```python
from build123d import *

# Parameters (mm, degrees)
SKETCH1_W           = 10
SKETCH1_H           = 10
BOSS_EXTRUDE1_DEPTH = 2.5
SKETCH2_R           = 0.75
SKETCH2_R_2         = 1
SKETCH2_R_3         = 1.25
SKETCH2_R_4         = 1.5
CUT_EXTRUDE1_DEPTH  = 24.468063405


with BuildPart() as part:
    # Sketch1 → Boss-Extrude1 (new body)
    with BuildSketch(Plane(origin=(0, 0, 0), x_dir=(1, 0, 0), z_dir=(0, 1, 0))):
        Rectangle(SKETCH1_W, SKETCH1_H)
        with BuildLine():
            Line((-5, -5), (-5, 5))
            Line((-5, 5), (-14.671400751, 5))
            ThreePointArc((-14.671400751, 5), (-15.5, 0), (-14.671400751, -5))
            Line((-14.671400751, -5), (-5, -5))
        make_face()
        with BuildLine():
            Line((-14.671400751, 5), (-5, 5))
            Line((-5, 5), (-5, 14.671400751))
            ThreePointArc((-5, 14.671400751), (-10.960155108, 10.960155108), (-14.671400751, 5))
        make_face()
        with BuildLine():
            Line((-5, 5), (5, 5))
            Line((5, 5), (5, 14.671400751))
            ThreePointArc((5, 14.671400751), (0, 15.5), (-5, 14.671400751))
            Line((-5, 14.671400751), (-5, 5))
        make_face()
        with BuildLine():
            Line((5, 5), (14.671400751, 5))
            ThreePointArc((14.671400751, 5), (10.960155108, 10.960155108), (5, 14.671400751))
            Line((5, 14.671400751), (5, 5))
        make_face()
        with BuildLine():
            ThreePointArc((15.5, 0), (15.291447146, 2.534096324), (14.671400751, 5))
            Line((14.671400751, 5), (5, 5))
            Line((5, 5), (5, -5))
            Line((5, -5), (14.671400751, -5))
            ThreePointArc((14.671400751, -5), (15.291447146, -2.534096324), (15.5, 0))
        make_face()
        with BuildLine():
            Line((16.5, -5), (16.5, 5))
            Line((16.5, 5), (14.671400751, 5))
            ThreePointArc((14.671400751, 5), (15.291447146, 2.534096324), (15.5, 0))
            ThreePointArc((15.5, 0), (15.291447146, -2.534096324), (14.671400751, -5))
            Line((14.671400751, -5), (16.5, -5))
        make_face()
        with BuildLine():
            ThreePointArc((5, -14.671400751), (10.960155108, -10.960155108), (14.671400751, -5))
            Line((14.671400751, -5), (5, -5))
            Line((5, -5), (5, -14.671400751))
        make_face()
        with BuildLine():
            Line((5, -14.671400751), (5, -5))
            Line((5, -5), (-5, -5))
            Line((-5, -5), (-5, -14.671400751))
            ThreePointArc((-5, -14.671400751), (0, -15.5), (5, -14.671400751))
        make_face()
        with BuildLine():
            Line((-5, -14.671400751), (-5, -5))
            Line((-5, -5), (-14.671400751, -5))
            ThreePointArc((-14.671400751, -5), (-10.960155108, -10.960155108), (-5, -14.671400751))
        make_face()
        with BuildLine():
            ThreePointArc((-14.671400751, -5), (-15.5, 0), (-14.671400751, 5))
            Line((-14.671400751, 5), (-16.5, 5))
            Line((-16.5, 5), (-16.5, -5))
            Line((-16.5, -5), (-14.671400751, -5))
        make_face()
        with BuildLine():
            Line((5, -16.5), (5, -14.671400751))
            ThreePointArc((5, -14.671400751), (0, -15.5), (-5, -14.671400751))
            Line((-5, -14.671400751), (-5, -16.5))
            Line((-5, -16.5), (5, -16.5))
        make_face()
        with BuildLine():
            ThreePointArc((-5, 14.671400751), (0, 15.5), (5, 14.671400751))
            Line((5, 14.671400751), (5, 16.5))
            Line((5, 16.5), (-5, 16.5))
            Line((-5, 16.5), (-5, 14.671400751))
        make_face()
    extrude(amount=BOSS_EXTRUDE1_DEPTH)

    # Sketch2 → Cut-Extrude1 (cut, through all)
    with BuildSketch(Plane(origin=(0, 2.5, 0), x_dir=(1, 0, 0), z_dir=(0, 1, 0))):
        with Locations(Location((0, 0, 0), (0, 0, 270))):
            Circle(SKETCH2_R)
        with Locations(Location((0, 3.75, 0), (0, 0, 270))):
            Circle(SKETCH2_R_2)
        with Locations(Location((0, 8, 0), (0, 0, 270))):
            Circle(SKETCH2_R_3)
        with Locations(Location((0, 12.75, 0), (0, 0, 270))):
            Circle(SKETCH2_R_4)
        with Locations(Location((3.247595264, 1.875, 0), (0, 0, 270))):
            Circle(SKETCH2_R_2)
        with Locations(Location((3.247595264, -1.875, 0), (0, 0, 270))):
            Circle(SKETCH2_R_2)
        with Locations(Location((0, -3.75, 0), (0, 0, 270))):
            Circle(SKETCH2_R_2)
        with Locations(Location((-3.247595264, -1.875, 0), (0, 0, 270))):
            Circle(SKETCH2_R_2)
        with Locations(Location((-3.247595264, 1.875, 0), (0, 0, 270))):
            Circle(SKETCH2_R_2)
        with Locations(Location((4, 6.92820323, 0), (0, 0, 270))):
            Circle(SKETCH2_R_3)
        with Locations(Location((6.92820323, 4, 0), (0, 0, 270))):
            Circle(SKETCH2_R_3)
        with Locations(Location((8, 0, 0), (0, 0, 270))):
            Circle(SKETCH2_R_3)
        with Locations(Location((6.92820323, -4, 0), (0, 0, 270))):
            Circle(SKETCH2_R_3)
        with Locations(Location((4, -6.92820323, 0), (0, 0, 270))):
            Circle(SKETCH2_R_3)
        with Locations(Location((0, -8, 0), (0, 0, 270))):
            Circle(SKETCH2_R_3)
        with Locations(Location((-4, -6.92820323, 0), (0, 0, 270))):
            Circle(SKETCH2_R_3)
        with Locations(Location((-6.92820323, -4, 0), (0, 0, 270))):
            Circle(SKETCH2_R_3)
        with Locations(Location((-8, 0, 0), (0, 0, 270))):
            Circle(SKETCH2_R_3)
        with Locations(Location((-6.92820323, 4, 0), (0, 0, 270))):
            Circle(SKETCH2_R_3)
        with Locations(Location((-4, 6.92820323, 0), (0, 0, 270))):
            Circle(SKETCH2_R_3)
        with Locations(Location((4.879213763, 11.77946404, 0), (0, 0, 270))):
            Circle(SKETCH2_R_4)
        with Locations(Location((9.01561146, 9.01561146, 0), (0, 0, 270))):
            Circle(SKETCH2_R_4)
        with Locations(Location((11.77946404, 4.879213763, 0), (0, 0, 270))):
            Circle(SKETCH2_R_4)
        with Locations(Location((12.75, 0, 0), (0, 0, 270))):
            Circle(SKETCH2_R_4)
        with Locations(Location((11.77946404, -4.879213763, 0), (0, 0, 270))):
            Circle(SKETCH2_R_4)
        with Locations(Location((9.01561146, -9.01561146, 0), (0, 0, 270))):
            Circle(SKETCH2_R_4)
        with Locations(Location((4.879213763, -11.77946404, 0), (0, 0, 270))):
            Circle(SKETCH2_R_4)
        with Locations(Location((0, -12.75, 0), (0, 0, 270))):
            Circle(SKETCH2_R_4)
        with Locations(Location((-4.879213763, -11.77946404, 0), (0, 0, 270))):
            Circle(SKETCH2_R_4)
        with Locations(Location((-9.01561146, -9.01561146, 0), (0, 0, 270))):
            Circle(SKETCH2_R_4)
        with Locations(Location((-11.77946404, -4.879213763, 0), (0, 0, 270))):
            Circle(SKETCH2_R_4)
        with Locations(Location((-12.75, 0, 0), (0, 0, 270))):
            Circle(SKETCH2_R_4)
        with Locations(Location((-11.77946404, 4.879213763, 0), (0, 0, 270))):
            Circle(SKETCH2_R_4)
        with Locations(Location((-9.01561146, 9.01561146, 0), (0, 0, 270))):
            Circle(SKETCH2_R_4)
        with Locations(Location((-4.879213763, 11.77946404, 0), (0, 0, 270))):
            Circle(SKETCH2_R_4)
    extrude(amount=-CUT_EXTRUDE1_DEPTH, mode=Mode.SUBTRACT)


solid = part.part
```
Here's how the part is built. I have some questions about the finished solid (model axes, mm). A direction names the side the tool comes from. Coordinates: 2 decimals unless noted, no trailing zeros. Order: outer loops, then holes, each group sorted by start corner. A loop starts at its lowest first (then second) coordinate and runs counter-clockwise, first axis right, second up.
Item 1: I need wall thicknesses on probe 1 along Z at (x, y) = (3, 1.7); probe 2 along X at (y, z) = (2.2, -6.5); probe 3 along X at (y, z) = (1.2, 0). Which ranges of each line are inside material? Lowest first, please.
Response values:
probe 1: z = -16.5 to -7.68, -6.18 to -2.84, -0.91 to 0.91, 2.84 to 6.18, 7.68 to 16.5
probe 2: x = -14.07 to -5.17, -2.83 to 2.83, 5.17 to 14.07
probe 3: x = -16.5 to -14.25, -11.25 to -9.25, -6.75 to -0.75, 0.75 to 6.75, 9.25 to 11.25, 14.25 to 16.5
Item 2: I'm going to push flat-ended pins straight in: pin 1 Ø1.5 at (y, z) = (2, 15.5) entering from -X; pin 2 Ø1.5 at (x, y) = (15.5, 1) entering from +Z; pin 3 Ø1.5 at (x, y) = (-15.5, 0.5) entering from -Z; pin 4 Ø1.8 at (x, z) = (-12.75, 0) entering from -Y. Where does each tip first touch, or does it pass through?
Response values:
pin 1: stops at x = -5
pin 2: stops at z = 5
pin 3: stops at z = -5
pin 4: passes through
Item 3: If we section it at C-C, the plane y = 0.8: Give the number of separate pieces and of enclosed holes in the cut face, then the cut area to 3 significant figures.
Response values:
separate pieces: 1
enclosed holes: 35
area: 613 mm2
Item 4: If we section it at A-A, the plane z = 0: List the corners of the cut face in (x, y) for me, then the cut area to 4 significant figures.
Response values:
outline: (-16.5, 0) - (-14.25, 0) - (-14.25, 2.5) - (-16.5, 2.5) - close; (-11.25, 0) - (-9.25, 0) - (-9.25, 2.5) - (-11.25, 2.5) - close; (-6.75, 0) - (-0.75, 0) - (-0.75, 2.5) - (-6.75, 2.5) - close; (0.75, 0) - (6.75, 0) - (6.75, 2.5) - (0.75, 2.5) - close; (9.25, 0) - (11.25, 0) - (11.25, 2.5) - (9.25, 2.5) - close; (14.25, 0) - (16.5, 0) - (16.5, 2.5) - (14.25, 2.5) - close
area: 51.25 mm2
Item 5: If we section it at B-B, the plane z = -12.75: List the corners of the cut face in (x, y) for me.
Response values:
outline: (-8.81, 0) - (-6.02, 0) - (-6.02, 2.5) - (-8.81, 2.5) - close; (-3.74, 0) - (-1.5, 0) - (-1.5, 2.5) - (-3.74, 2.5) - close; (1.5, 0) - (3.74, 0) - (3.74, 2.5) - (1.5, 2.5) - close; (6.02, 0) - (8.81, 0) - (8.81, 2.5) - (6.02, 2.5) - close
Item 6: Thinking about a two-plate mould opening in Z: for faces 4 (the face through (-16, 1, -5)), 5 (the face through (-16, 1, 5)), 6 (the face through (-12.3, 1.27, 1.43)), which applies, pulls with the +Z half, pulls with the -Z half, needs draft (parallel to the pull), parting line crosses it, or undercut?
Response values:
face 4: pulls with the -Z half
face 5: pulls with the +Z half
face 6: undercut
Item 7: Which directions (+Z, -Z, +X, -X, +Y, -Y) give clear straight access to the entire face, cutting with the end or side of a thin tool? Please do faces 1 (the face through (16, 1, 5)), 2 (the face through (0.07, 1.27, 11.25)), 3 (the face through (16, 1, -5)).
Response values:
face 1: +Z, +X, +Y, -Y
face 2: +Y, -Y
face 3: -Z, +X, +Y, -Y
